from build123d import *

# Parameters (mm, degrees)
SKETCH1_W            = 101.6
SKETCH1_H            = 50.8
BOSS_EXTRUDE1_DEPTH  = 38.608
CUT_EXTRUDE1_DEPTH   = 69.67588852
MIRROR2_COPY_1_DEPTH = 69.67588852


with BuildPart() as part:
    # Sketch1 → Boss-Extrude1 (new body)
    with BuildSketch(Plane.XY):
        Rectangle(SKETCH1_W, SKETCH1_H)
    extrude(amount=BOSS_EXTRUDE1_DEPTH)

    # Sketch4 → Cut-Extrude1 (cut, through all)
    with BuildSketch(Plane.XY.offset(38.608)):
        with BuildLine():
            Line((47.3075, 23.8125), (47.9425, 23.8125))
            ThreePointArc((47.9425, 23.8125), (49.53, 22.225), (47.9425, 20.6375))
            Line((47.9425, 20.6375), (47.3075, 20.6375))
            ThreePointArc((47.3075, 20.6375), (45.72, 22.225), (47.3075, 23.8125))
        make_face()
    cut_extrude1 = extrude(amount=-CUT_EXTRUDE1_DEPTH, mode=Mode.SUBTRACT)

    # Mirror1: Cut-Extrude1 across plane
    add(cut_extrude1.mirror(Plane.ZX), mode=Mode.SUBTRACT)

    # Mirror2: Cut-Extrude1 across plane
    add(cut_extrude1.mirror(Plane(origin=(0, 0, 0), x_dir=(0, 0, 1), z_dir=(1, 0, 0))), mode=Mode.SUBTRACT)

    # Mirror2 copy 1 sketch → Mirror2 copy 1 (cut, through all)
    with BuildSketch(Plane(origin=(0, 0, 38.608), x_dir=(-1, 0, 0), z_dir=(0, 0, 1))):
        with BuildLine():
            Line((47.3075, 23.8125), (47.9425, 23.8125))
            ThreePointArc((47.9425, 23.8125), (49.53, 22.225), (47.9425, 20.6375))
            Line((47.9425, 20.6375), (47.3075, 20.6375))
            ThreePointArc((47.3075, 20.6375), (45.72, 22.225), (47.3075, 23.8125))
        make_face()
    extrude(amount=-MIRROR2_COPY_1_DEPTH, mode=Mode.SUBTRACT)


solid = part.part
CAD build for the part. Positions are in the model's coordinates, mm. A direction names the side the tool comes from. Give positions to 0.01 mm unless a question says otherwise; leave off trailing zeros. Order: outer loops, then holes, each group sorted by start corner. A loop starts at its lowest first (then second) coordinate and runs counter-clockwise, first axis right, second up. Notation, with made-up numbers: (53, 78) - (104, 78) arc R19 ccw to (104, 91) - close; hole circle Ø5 at (-20, 11). An arc over 180 degrees is marked (long way). Write each question's results on one line, items separated by ' | '.
1. 3-axis set-ups, long thin cutter, end or side, ignore diameter. For faces 4 (the face through (-50.8, 0, 19)), 5 (the face through (45.72, 22.19, 19.57)): which of +Z, -Z, +X, -X, +Y, -Y reach the whole face in a straight line?
Calculated:
face 4: +Z, -Z, -X, +Y, -Y | face 5: +Z, -Z
2. Pull direction X, two halves, no side cores. Call faces 1 (the face through (50.8, 0, 19)), 2 (the face through (-45.72, -22.19, 19.57)), 3 (the face through (-1, 0, 38.608)): released by +X, released by -X, zero draft, split by the parting line, or undercut.
Calculated:
face 1: released by +X | face 2: undercut | face 3: zero draft
3. Saw through at A-A on y = -22. List the corners of the cut face in (x, z), and give its area (3 significant figures).
Calculated:
outline: (-50.8, 0) - (-49.51, 0) - (-49.51, 38.61) - (-50.8, 38.61) - close; (-45.74, 0) - (45.74, 0) - (45.74, 38.61) - (-45.74, 38.61) - close; (49.51, 0) - (50.8, 0) - (50.8, 38.61) - (49.51, 38.61) - close | area: 3,630 mm2
